from build123d import *

# Parameters (mm, degrees)
SKETCH1_W           = 36
SKETCH1_H           = 12
SKETCH1_R           = 2.1
BOSS_EXTRUDE1_DEPTH = 12
SKETCH1_2_R         = 2.1
BOSS_EXTRUDE2_DEPTH = 2


with BuildPart() as part:
    # Sketch1 → Boss-Extrude1 (new body)
    with BuildSketch(Plane(origin=(0, 0, 0), x_dir=(1, 0, 0), z_dir=(0, 1, 0))):
        Rectangle(SKETCH1_W, SKETCH1_H)
        with Locations(Location((0, 0, 0), (0, 0, 270))):
            Circle(SKETCH1_R, mode=Mode.SUBTRACT)
        with Locations(Location((-12, 0, 0), (0, 0, 270))):
            Circle(SKETCH1_R, mode=Mode.SUBTRACT)
        with Locations(Location((12, 0, 0), (0, 0, 270))):
            Circle(SKETCH1_R, mode=Mode.SUBTRACT)
    extrude(amount=BOSS_EXTRUDE1_DEPTH)

    # Sketch1_2 → Boss-Extrude2 (add)
    with BuildSketch(Plane(origin=(0, 0, 0), x_dir=(1, 0, 0), z_dir=(0, 1, 0))):
        with Locations(Location((-12, 0, 0), (0, 0, 270))):
            Circle(SKETCH1_2_R)
        with Locations(Location((0, 0, 0), (0, 0, 270))):
            Circle(SKETCH1_2_R)
        with Locations(Location((12, 0, 0), (0, 0, 270))):
            Circle(SKETCH1_2_R)
    extrude(amount=BOSS_EXTRUDE2_DEPTH)


solid = part.part
For this review, take the finished solid that the model builds, in its own axes (mm). A direction names the side the tool comes from. Coordinates: 2 decimals unless noted, no trailing zeros. Order: outer loops, then holes, each group sorted by start corner. A loop starts at its lowest first (then second) coordinate and runs counter-clockwise, first axis right, second up. Notation, with made-up numbers: (1.5, 82.5) - (35.5, 82.5) arc R26 cw to (35.5, 110.5) - close; hole circle Ø7 at (82.5, 66). An arc over 180 degrees is marked (long way). Answer as CSV lines item,"result". Start each with the question number.
1) Add section D-D (z = -1.75). State the section outline as (x, y) points, then the cut area to 3 significant figures.
2) Add section C-C (y = 10.25). State the section outline as (x, z) points, then the cut area to 3 significant figures.
3) To check wall thickness, follow line 1 along X through (y, z) = (5, 0); line 2 along X through (y, z) = (5.75, 1.75); line 3 along Z through (x, y) = (-0.5, 8.25). State the ranges of each line that lie inside material, in increasing order. Write a range as [from, to].
4) Draft analysis for pull direction X (two halves, no side actions). For faces 3 (the flat face through (-18, 6, 0)), 4 (the flat face through (0, 0, 0)), 5 (the cylindrical face through (13.77, 6.93, 1.13)), 6 (the cylindrical face through (0.631, 6.93, 2.003)), state which applies: +X half, -X half, draft (parallel to the pull), parting line (faces both ways), or undercut.
5) Add section A-A (x = -12). State the section outline as (y, z) points.
6) Add section B-B (z = 0). State the section outline as (x, y) points, then the cut area to 3 significant figures.
7) Machinability: for faces 1 (the flat face through (0, 6, 6)), 2 (the flat face through (-12, 2, 0)), which of the approach directions +Z, -Z, +X, -X, +Y, -Y give a long, thin tool a straight path to every point of the face, cutting with its end or side? Answer none if there is none.
8) Insertion check: P1, Ø3.5, axis at x = -0.5, z = -0.5, coming from the +Y side; P2, Ø1.3, axis at x = -12, z = -0.5, coming from the +Y side. Each pin has a flat end and moves straight along its axis. Give the tip position at first contact, or say it passes through.
Result:
1,outline,"(-18, 0) - (18, 0) - (18, 12) - (13.16, 12) - (13.16, 2) - (10.84, 2) - (10.84, 12) - (1.16, 12) - (1.16, 2) - (-1.16, 2) - (-1.16, 12) - (-10.84, 12) - (-10.84, 2) - (-13.16, 2) - (-13.16, 12) - (-18, 12) - close"
1,area,"362 mm^2"
2,outline,"(-18, -6) - (18, -6) - (18, 6) - (-18, 6) - close; hole circle Ø4.2 at (-12, 0); hole circle Ø4.2 at (0, 0); hole circle Ø4.2 at (12, 0)"
2,area,"390 mm^2"
3,line 1,"[-18, -14.1], [-9.9, -2.1], [2.1, 9.9], [14.1, 18]"
3,line 2,"[-18, -13.16], [-10.84, -1.16], [1.16, 10.84], [13.16, 18]"
3,line 3,"[-6, -2.04], [2.04, 6]"
4,face 3,"-X half"
4,face 4,"draft"
4,face 5,"undercut"
4,face 6,"undercut"
5,outline,"(0, -6) - (12, -6) - (12, -2.1) - (2, -2.1) - (2, 2.1) - (12, 2.1) - (12, 6) - (0, 6) - close"
6,outline,"(-18, 0) - (18, 0) - (18, 12) - (14.1, 12) - (14.1, 2) - (9.9, 2) - (9.9, 12) - (2.1, 12) - (2.1, 2) - (-2.1, 2) - (-2.1, 12) - (-9.9, 12) - (-9.9, 2) - (-14.1, 2) - (-14.1, 12) - (-18, 12) - close"
6,area,"306 mm^2"
7,face 1,"+Z, +X, -X, +Y, -Y"
7,face 2,"+Y"
8,P1,"y = 12"
8,P2,"y = 2"
